```python
from build123d import *
from build123d.topology import SkipClean

# Parameters (mm, degrees)
SKETCH1_R           = 49
BOSS_EXTRUDE1_DEPTH = 25.5
SKETCH2_R           = 39.95
BOSS_EXTRUDE2_DEPTH = 1.5
DOME1_FACE_RADIUS   = 39.95
DOME1_HEIGHT        = 20
CHAMFER1_SIZE       = 8
CHAMFER1_SIZE_2     = 10.811379504
SKETCH3_R           = 12
BOSS_EXTRUDE3_DEPTH = 60


with BuildPart() as part:
    # Sketch1 → Boss-Extrude1 (new body)
    with BuildSketch(Plane(origin=(0, 0, 0), x_dir=(1, 0, 0), z_dir=(0, 1, 0))):
        with Locations(Location((0, 0, 0), (0, 0, 270))):
            Circle(SKETCH1_R)
    extrude(amount=BOSS_EXTRUDE1_DEPTH)

    # Sketch2 → Boss-Extrude2 (add)
    with BuildSketch(Plane(origin=(0, 25.5, 0), x_dir=(1, 0, 0), z_dir=(0, 1, 0))):
        with Locations(Location((0, 0, 0), (0, 0, 270))):
            Circle(SKETCH2_R)
    extrude(amount=BOSS_EXTRUDE2_DEPTH)

    # Dome1: a dome of height H over a round flat face of radius A is a cap of a sphere of radius (A * A + H * H) / (2 * H)
    dome1_r = (DOME1_FACE_RADIUS * DOME1_FACE_RADIUS + DOME1_HEIGHT * DOME1_HEIGHT) / (2 * DOME1_HEIGHT)
    dome1_base = Plane((0, 27, 0), z_dir=(0, 1, 0))
    with Locations(dome1_base.offset(DOME1_HEIGHT - dome1_r)):
        dome1_ball = Sphere(dome1_r, mode=Mode.PRIVATE)
    add(split(dome1_ball, bisect_by=dome1_base, keep=Keep.TOP, mode=Mode.PRIVATE))

    # Chamfer1
    # the kernel refuses this chamfer: 10.811379504, 8 mm, written as the material it takes off along each edge
    with BuildSketch(Plane(origin=(0, 25.5, 0), x_dir=(0, 0, 1), z_dir=(-1, 0, 0))) as chamfer1_piece_1_section:
        Polygon((49, -CHAMFER1_SIZE), (49 - CHAMFER1_SIZE_2, 0), (49, 0), align=None)
    chamfer1_piece_1 = revolve(axis=Axis((0, 25.5, 0), (0, 1, 0)), mode=Mode.PRIVATE)
    chamfer1_piece_1 = chamfer1_piece_1 - Plane(origin=(0, 20.910194106, 0), x_dir=(0, 0, 1), z_dir=(0, -1, 0)) * Cylinder(39.95, 196, mode=Mode.PRIVATE)
    add(chamfer1_piece_1, mode=Mode.SUBTRACT)

    # Sketch3 → Boss-Extrude3 (add)
    with SkipClean():  # the faces are left unmerged after this step: merging them gives an invalid solid
        with BuildSketch(Plane.XZ):
            with Locations(Location((0, 0, 0), (0, 0, 270))):
                Circle(SKETCH3_R)
        extrude(amount=BOSS_EXTRUDE3_DEPTH)


solid = part.part
```
Verification items for the finished model (mm, model axes). A direction names the side the tool comes from. Round coordinates to 2 decimals unless told otherwise and drop trailing zeros. Write each loop counter-clockwise with the first axis right and the second up, starting at its lowest first coordinate (ties: lowest second). Pieces come first, ordered by that corner, then holes. Notation, with made-up numbers: (18.25, 56) - (76.25, 56) arc R25 ccw to (76.25, 71) - close; hole circle Ø9 at (-37.5, 53.5). An arc over 180 degrees is marked (long way). Answer as a JSON object with one key per item and string values. Group by question number.
Q1. Thickness scan on line 1 (Y direction, x = -24, z = 41); line 2 (Y direction, x = 36, z = 4); line 3 (X direction, y = -19.5, z = 7). Record the ranges inside material, lowest first.
Q2. Go/stop test with flat-tipped pins: pin 1 Ø1 at (x, z) = (-4.5, -12) entering from -Y; pin 2 Ø3 at (x, y) = (-31.5, 20.5) entering from -Z; pin 3 Ø10 at (x, z) = (28, -17) entering from +Y. Record where each tip stops, or that it passes through.
Q3. Section check C-C, the plane y = 15. Enter the section's corners in (x, z), plus the area to 3 significant figures.
Q4. Tool access check on faces 1 (the cylindrical face through (14.718, 8.628, 46.737)), 2 (the flat face through (-10, 0, 10)). Record the directions out of +Z, -Z, +X, -X, +Y, -Y that give a thin tool (end or side, any length) a straight path to the whole face; none if there is none.
Q5. Section check D-D, the plane y = -20.5. Enter the section's corners in (x, z).
Q6. Section check B-B, the plane z = 0. Enter the section's corners in (x, y), plus the area to 3 significant figures.
Q7. Section check A-A, the plane x = 0. Enter the section's corners in (y, z).
Found:
{
 "1": {"line 1": "y = 0 to 18.6", "line 2": "y = 0 to 31.42", "line 3": "x = -9.75 to 9.75"},
 "2": {"pin 1": "stops at y = 0", "pin 2": "stops at z = -35.16", "pin 3": "stops at y = 38.57"},
 "3": {"outline": "circle Ø98 at (0, 0)", "area": "7,540 mm^2"},
 "4": {"face 1": "+Y, -Y", "face 2": "-Y"},
 "5": {"outline": "circle Ø24 at (0, 0)"},
 "6": {"outline": "(-49, 0) - (-12, 0) - (-12, -60) - (12, -60) - (12, 0) - (49, 0) - (49, 17.5) - (39.95, 24.2) - (39.95, 27) arc R49.9 ccw to (-39.95, 27) - (-39.95, 24.2) - (-49, 17.5) - close", "area": "5,090 mm^2"},
 "7": {"outline": "(-60, -12) - (0, -12) - (0, -49) - (17.5, -49) - (24.2, -39.95) - (27, -39.95) arc R49.9 ccw to (27, 39.95) - (24.2, 39.95) - (17.5, 49) - (0, 49) - (0, 12) - (-60, 12) - close"}
}
